from build123d import *

# Parameters (mm, degrees)
SKETCH2_W               = 116.84
SKETCH2_H               = 33.02
BOSS_EXTRUDE1_DEPTH     = 2.54
SKETCH3_W               = 6.35
SKETCH3_H               = 33.02
BOSS_EXTRUDE2_DEPTH     = 25.4
CUT_EXTRUDE1_DEPTH      = 125.589524439
CUT_EXTRUDE1_DEPTH_BACK = 125.589524439
SKETCH4_R               = 3.175
SKETCH5_W               = 116.84
SKETCH5_H               = 2.54
BOSS_EXTRUDE3_DEPTH     = 50.8
SKETCH6_W               = 6.35
SKETCH6_H               = 35.052
BOSS_EXTRUDE4_DEPTH     = 7.62
SKETCH7_W               = 35.052
SKETCH7_H               = 4.826
BOSS_EXTRUDE5_DEPTH     = 6.35
SKETCH8_W               = 35.052
SKETCH8_H               = 4.826
BOSS_EXTRUDE6_DEPTH     = 6.35
FILLET1_R               = 2.54
FILLET7_R               = 2.54
FILLET8_R               = 2.54
CUT_EXTRUDE2_REACH      = 137.652
SKETCH16_W              = 19.05
SKETCH16_H              = 40.894


with BuildPart() as part:
    # Sketch2 → Boss-Extrude1 (new body)
    with BuildSketch(Plane(origin=(0, 0, 0), x_dir=(1, 0, 0), z_dir=(0, 1, 0))):
        with Locations((58.42, 16.51)):
            Rectangle(SKETCH2_W, SKETCH2_H)
    extrude(amount=BOSS_EXTRUDE1_DEPTH)

    # Sketch3 → Boss-Extrude2 (add)
    with BuildSketch(Plane(origin=(0, 2.54, 0), x_dir=(1, 0, 0), z_dir=(0, 1, 0))):
        with Locations((3.175, 16.51)):
            Rectangle(SKETCH3_W, SKETCH3_H)
        with Locations((113.665, 16.51)):
            Rectangle(SKETCH3_W, SKETCH3_H)
    extrude(amount=BOSS_EXTRUDE2_DEPTH)

    # Sketch4 → Cut-Extrude1 (cut, two sides: drawn at the far end of the back side and taken through both)
    with BuildSketch(Plane.ZY.offset(-CUT_EXTRUDE1_DEPTH_BACK)):
        with Locations((-16.51, 18.93000799)):
            Circle(SKETCH4_R)
    extrude(amount=CUT_EXTRUDE1_DEPTH + CUT_EXTRUDE1_DEPTH_BACK, mode=Mode.SUBTRACT)

    # Sketch5 → Boss-Extrude3 (add)
    with BuildSketch(Plane.XY):
        with Locations((58.42, 1.27)):
            Rectangle(SKETCH5_W, SKETCH5_H)
    extrude(amount=BOSS_EXTRUDE3_DEPTH)

    # Sketch6 → Boss-Extrude4 (add)
    with BuildSketch(Plane(origin=(0, 2.54, 0), x_dir=(1, 0, 0), z_dir=(0, 1, 0))):
        with Locations((3.175, -23.622)):
            Rectangle(SKETCH6_W, SKETCH6_H)
        with Locations((113.665, -23.622)):
            Rectangle(SKETCH6_W, SKETCH6_H)
    extrude(amount=BOSS_EXTRUDE4_DEPTH)

    # Sketch7 → Boss-Extrude5 (add)
    with BuildSketch(Plane.ZY):
        with Locations((23.622, 7.747)):
            Rectangle(SKETCH7_W, SKETCH7_H)
    extrude(amount=BOSS_EXTRUDE5_DEPTH)

    # Sketch8 → Boss-Extrude6 (add)
    with BuildSketch(Plane(origin=(116.84, 0, 0), x_dir=(0, 0, -1), z_dir=(1, 0, 0))):
        with Locations((-23.622, 7.747)):
            Rectangle(SKETCH8_W, SKETCH8_H)
    extrude(amount=BOSS_EXTRUDE6_DEPTH)

    # Fillet1
    fillet1_edges = [part.edges().sort_by_distance(p)[0] for p in [
        (6.35, 2.54, -16.51),
        (6.35, 15.24, 0),
        (6.35, 15.24, -33.02),
        (3.175, 27.94, 0),
        (3.175, 27.94, -33.02),
        (58.42, 2.54, -33.02),
        (110.49, 2.54, -16.51),
        (110.49, 15.24, -33.02),
        (110.49, 15.24, 0),
        (113.665, 27.94, 0),
        (113.665, 27.94, -33.02),
        (3.175, 2.54, 0),
        (113.665, 2.54, 0),
        (3.175, 2.54, 41.148),
        (6.35, 2.54, 23.622),
        (6.35, 6.35, 41.148),
        (3.175, 2.54, 6.096),
        (6.35, 6.35, 6.096),
        (6.35, 10.16, 23.622),
        (113.665, 2.54, 6.096),
        (110.49, 2.54, 23.622),
        (110.49, 6.35, 6.096),
        (113.665, 2.54, 41.148),
        (110.49, 6.35, 41.148),
        (110.49, 10.16, 23.622),
    ]]
    fillet(fillet1_edges, radius=FILLET1_R - 0.0001)  # a hair under: the kernel refuses the full size

    # Fillet7
    fillet7_edges = [part.edges().sort_by_distance(p)[0] for p in [
        (0, 1.27, 50.8),
        (116.84, 1.27, 50.8),
    ]]
    fillet(fillet7_edges, radius=FILLET7_R)

    # Fillet8
    fillet8_edges = [part.edges().sort_by_distance(p)[0] for p in [
        (116.84, 5.20695, 41.148),
        (116.84, 3.283919486, 41.891919486),
        (116.84, 2.54, 45.97395),
        (116.096051224, 2.54, 50.056051224),
        (0, 5.20695, 41.148),
        (0, 3.283919486, 41.891919486),
        (0, 2.54, 45.97395),
        (0.743948776, 2.54, 50.056051224),
        (58.42, 2.54, 50.8),
    ]]
    fillet(fillet8_edges, radius=FILLET8_R - 0.0001)  # a hair under: the kernel refuses the full size

    # Sketch16 → Cut-Extrude2 (cut, up to next)
    with BuildSketch(Plane(origin=(0, 2.54, 0), x_dir=(1, 0, 0), z_dir=(0, 1, 0)), mode=Mode.PRIVATE) as cut_extrude2_sk1:
        with Locations((58.42, -7.62)):
            Rectangle(SKETCH16_W, SKETCH16_H)
    cut_extrude2_tool1 = extrude(cut_extrude2_sk1.sketch, amount=-CUT_EXTRUDE2_REACH, mode=Mode.PRIVATE) & part.part
    add(cut_extrude2_tool1.solids().sort_by_distance((58.42, 2.54, 7.62))[0], mode=Mode.SUBTRACT)


solid = part.part
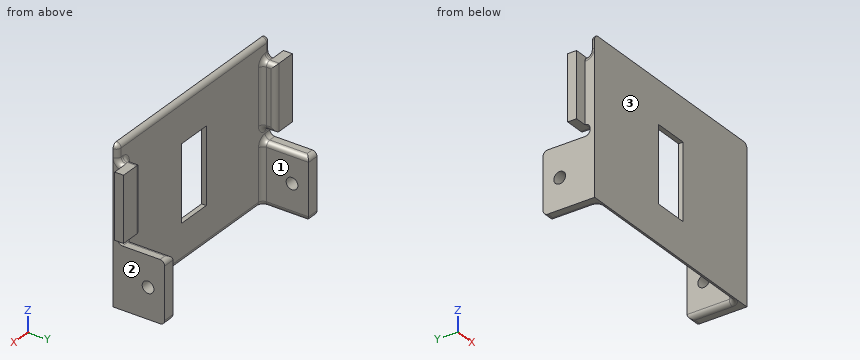
Geometry check sheet. Reference: the model listing, model coordinates, mm. Face numbers are marked on the shaded views. Give positions to 0.01 mm unless a question says otherwise; leave off trailing zeros. Write each loop counter-clockwise with the first axis right and the second up, starting at its lowest first coordinate (ties: lowest second). Pieces come first, ordered by that corner, then holes. Notation, with made-up numbers: (-14.75, -24.75) - (-7.75, -24.75) arc R11 ccw to (-7.75, -19.75) - close; hole circle Ø2 at (-40, 89). An arc over 180 degrees is marked (long way). Put each result on its own line as item: value.
1. Sectioned sample at D-D, the plane z = 21. Enter the section's corners in (x, y) (3 decimals), plus the area to 3 significant figures.
Ans:
outline: (-6.35, 5.334) - (0, 5.334) - (0, 0) - (48.895, 0) - (48.895, 2.54) - (8.89, 2.54) arc R2.54 cw to (6.35, 5.08) - (6.35, 7.62) arc R2.54 ccw to (3.81, 10.16) - (-6.35, 10.16) - close; (67.945, 0) - (116.84, 0) - (116.84, 5.334) - (123.19, 5.334) - (123.19, 10.16) - (113.03, 10.16) arc R2.54 ccw to (110.49, 7.62) - (110.49, 5.08) arc R2.54 cw to (107.95, 2.54) - (67.945, 2.54) - close
area: 406 mm²
2. Thickness scan on line 1 (Y direction, x = 113, z = -16.51) (3 decimals); line 2 (X direction, y = 5.5, z = -14); line 3 (Y direction, x = 86, z = 34). Record the ranges inside material, lowest first.
Ans:
line 1: y = 0 to 15.755, 22.105 to 27.94
line 2: x = 0 to 6.35, 110.49 to 116.84
line 3: y = 0 to 2.54
3. Sectioned sample at B-B, the plane z = -16.51. Enter the section's corners in (x, y) (3 decimals), plus the area to 3 significant figures.
Ans:
outline: (0, 0) - (116.84, 0) - (116.84, 15.755) - (110.49, 15.755) - (110.49, 5.08) arc R2.54 cw to (107.95, 2.54) - (8.89, 2.54) arc R2.54 cw to (6.35, 5.08) - (6.35, 15.755) - (0, 15.755) - close; (0, 22.105) - (6.35, 22.105) - (6.35, 27.94) - (0, 27.94) - close; (110.49, 22.105) - (116.84, 22.105) - (116.84, 27.94) - (110.49, 27.94) - close
area: 541 mm²
4. Draft check along X on the marked faces 1, 2 and 3. Enter one of: +X half, -X half, draft (parallel to the pull), parting line (faces both ways), or undercut.
Ans:
face 1: undercut
face 2: +X half
face 3: draft
5. Sectioned sample at A-A, the plane y = 14.5. Enter the section's corners in (x, z), plus the area to 3 significant figures.
Ans:
outline: (0, -33.02) - (3.81, -33.02) arc R2.54 ccw to (6.35, -30.48) - (6.35, -2.54) arc R2.54 ccw to (3.81, 0) - (0, 0) - close; (110.49, -30.48) arc R2.54 ccw to (113.03, -33.02) - (116.84, -33.02) - (116.84, 0) - (113.03, 0) arc R2.54 ccw to (110.49, -2.54) - close
area: 414 mm²
6. Go/stop test with flat-tipped pins: pin 1 (11 mm diameter, centred on x = 120.5, z = 30, fed in from +Y); pin 2 (3 mm diameter, centred on x = 115.5, y = 13.5, fed in from +Z); pin 3 (5.5 mm diameter, centred on x = -3, y = 7, fed in from -Z). Record where each tip stops, or that it passes through.
Ans:
pin 1: stops at y = 10.16
pin 2: stops at z = 0
pin 3: stops at z = 6.1
